Check sheet for the modelled part. Datum: model origin and axes. Units: mm. A direction names the side the tool comes from. Give positions to 0.01 mm unless a question says otherwise; leave off trailing zeros. Write each loop counter-clockwise with the first axis right and the second up, starting at its lowest first coordinate (ties: lowest second). Pieces come first, ordered by that corner, then holes.
from build123d import *

# Parameters (mm, degrees)
BOSS_EXTRUDE1_DEPTH       = 103
BOSS_EXTRUDE2_DEPTH       = 5
CUT_EXTRUDE1_DEPTH        = 120.616052434
CUT_EXTRUDE1_DEPTH_BACK   = 5
M5_CLEARANCE_HOLE1_REACH  = 162.532
M5_CLEARANCE_HOLE1_BORE_R = 1.5


with BuildPart() as part:
    # Sketch1 → Boss-Extrude1 (new body)
    with BuildSketch(Plane.XY):
        with BuildLine():
            Line((2.925360851, 74.488852712), (80.707106781, -3.292893219))
            ThreePointArc((80.707106781, -3.292893219), (80.923879533, -4.382683432), (80, -5))
            Line((80, -5), (0, -5))
            Line((0, -5), (0, 0))
            Line((0, 0), (53.443650814, 0))
            ThreePointArc((53.443650814, 0), (59.910807541, 4.321215973), (58.393398282, 11.949747468))
            Line((58.393398282, 11.949747468), (-0.610173055, 70.953318806))
            Line((-0.610173055, 70.953318806), (2.925360851, 74.488852712))
        make_face()
    extrude(amount=BOSS_EXTRUDE1_DEPTH)

    # Sketch2 → Boss-Extrude2 (add)
    with BuildSketch(Plane(origin=(38.707106781, 38.707106781, 0), x_dir=(0, 0, -1), z_dir=(0.7071067811865487, 0.7071067811865465, 0))):
        Polygon((-61.518289963, -48.391918986), (-100.409162928, -9.501046021), (-103, -6.910208949), (-103, -9.738636074), (-61.518289963, -51.220346111), (0, 10.297943853), (0, 13.126370977), (-1.414213562, 11.712157415), align=None)
    extrude(amount=BOSS_EXTRUDE2_DEPTH)

    # Sketch4 → Cut-Extrude1 (cut, two sides)
    with BuildSketch(Plane(origin=(38.707106781, 38.707106781, 0), x_dir=(0, 0, -1), z_dir=(0.7071067811865487, 0.7071067811865465, 0))) as cut_extrude1_sk:
        Polygon((-287.389423781, -191.29963273), (-103, -6.910208949), (-45.486760671, 50.60303038), (138.902663111, 234.992454162), (-229.876184452, 603.771301725), (-656.168271344, 177.479214832), align=None)
    extrude(amount=CUT_EXTRUDE1_DEPTH, mode=Mode.SUBTRACT)
    extrude(cut_extrude1_sk.sketch, amount=-CUT_EXTRUDE1_DEPTH_BACK, mode=Mode.SUBTRACT)

    # M5 Clearance Hole1 bore → M5 Clearance Hole1 (cut, up to next)
    with BuildSketch(Plane(origin=(80.628758112, -3.214544549, 114.598480766), x_dir=(-0.4999999999999967, 0.4999999999999984, 0.707106781186551), z_dir=(0.7071067811865487, 0.7071067811865464, 0)), mode=Mode.PRIVATE) as m5_clearance_hole1_sk1:
        with Locations((-0.829965603, -69.236760125)):
            Circle(M5_CLEARANCE_HOLE1_BORE_R)
    m5_clearance_hole1_tool1 = extrude(m5_clearance_hole1_sk1.sketch, amount=-M5_CLEARANCE_HOLE1_REACH, mode=Mode.PRIVATE) & part.part
    # M5 Clearance Hole1 bore → M5 Clearance Hole1 (cut, up to next)
    with BuildSketch(Plane(origin=(80.628758112, -3.214544549, 114.598480766), x_dir=(-0.4999999999999967, 0.4999999999999984, 0.707106781186551), z_dir=(0.7071067811865487, 0.7071067811865464, 0)), mode=Mode.PRIVATE) as m5_clearance_hole1_sk2:
        with Locations((-0.829965603, -109.236760125)):
            Circle(M5_CLEARANCE_HOLE1_BORE_R)
    m5_clearance_hole1_tool2 = extrude(m5_clearance_hole1_sk2.sketch, amount=-M5_CLEARANCE_HOLE1_REACH, mode=Mode.PRIVATE) & part.part
    add(m5_clearance_hole1_tool1.solids().sort_by_distance((46.425361, 30.988853, 65.053824))[0], mode=Mode.SUBTRACT)
    add(m5_clearance_hole1_tool2.solids().sort_by_distance((26.425361, 50.988853, 36.769553))[0], mode=Mode.SUBTRACT)


solid = part.part
1) Access from +Z, -Z, +X, -X, +Y, -Y to the whole of each face (thin tool, end or side, straight path). Record for faces 1 (the flat face through (0, -3, 51)), 2 (the flat face through (60.208, 20.693, 81.969)), 3 (the flat face through (55.223, 25.677, 31.19)), 4 (the flat face through (35.861, 34.483, 39.335)).
2) Scan lines: L1, parallel to Y at x = 20, z = 14.5; L2, parallel to Y at x = 12.5, z = 37.5; L3, parallel to Z at x = 60, y = 20. Record each from-to range of solid material in increasing order.
3) Gauge pin test, flat ends, axial feed: pin 1 (5 mm diameter, centred on y = 48, z = 84.5, fed in from -X); pin 2 (4 mm diameter, centred on x = 66.5, z = 65, fed in from +Y); pin 3 (3 mm diameter, centred on x = 26, z = 82.5, fed in from +Y). Record the tip position at first contact, or that the pin passes through.
4) Sectioned sample at D-D on y = 42. Record the boundary of the cut face in (x, z).
5) Sectioned sample at B-B on z = 80. Record the boundary of the cut face in (x, y).
6) Sectioned sample at C-C on x = 24. Give the number of separate pieces and of enclosed holes in the cut face, then the cut area to 3 significant figures.
7) Sectioned sample at A-A on x = 36.5. Record the boundary of the cut face in (y, z).
8) Draft check along Z on faces 5 (the flat face through (52.614, 28.286, 30.329)), 6 (the flat face through (65.716, 18.769, 44.111)), 7 (the cylindrical face through (24.821, 49.107, 35.282)), 8 (the flat face through (50, -1, 103)). Enter one of: +Z half, -Z half, draft (parallel to the pull), parting line (faces both ways), or undercut.
Answers below:
1. face 1: +Z, -Z, -X, -Y
1. face 2: +Y
1. face 3: -Z, +X
1. face 4: +Z, -Z, -X
2. L1: y = -5 to 0, 50.34 to 57.41
2. L2: y = -5 to 0, 57.84 to 64.91
2. L3: z = 38.58 to 41.41, 81.63 to 84.45
3. pin 1: stops at x = 27.28
3. pin 2: stops at y = 12.91
3. pin 3: stops at y = 47.82
4. outline: (28.34, 0) - (35.41, 0) - (35.41, 5.64) - (42.49, 10.64) - (42.49, 13.47) - (35.41, 8.47) - (35.41, 91.43) - (28.34, 86.43) - close
5. outline: (0, -5) - (80, -5) arc R1 ccw to (80.71, -3.29) - (61.86, 15.56) - (65.39, 19.09) - (63.39, 21.09) - (59.86, 17.56) - (27.33, 50.08) - (23.79, 46.55) - (58.39, 11.95) arc R7 cw to (53.44, 0) - (0, 0) - close
6. separate pieces: 2
6. enclosed holes: 1
6. area: 1,060 mm2
7. outline: (-5, 0) - (0, 0) - (0, 103) - (-5, 103) - close; (33.84, 0) - (40.91, 0) - (40.91, 7.18) - (47.99, 2.18) - (47.99, 5.01) - (40.91, 10.01) - (40.91, 92.97) - (33.84, 97.97) - close
8. face 5: undercut
8. face 6: draft
8. face 7: undercut
8. face 8: +Z half
